Design review of the part built by this model. Coordinates are the model's own, in mm. A direction names the side the tool comes from. Coordinates: 2 decimals unless noted, no trailing zeros. Write each loop counter-clockwise with the first axis right and the second up, starting at its lowest first coordinate (ties: lowest second). Pieces come first, ordered by that corner, then holes. Notation, with made-up numbers: (3, 19) - (62, 19) arc R18 cw to (62, 30) - close; hole circle Ø7 at (85, 88). An arc over 180 degrees is marked (long way). One line per item, written item: value.
Autodesk Inventor part; units mm, degrees
ref_plane "YZ Plane" through (0, 0, 0) normal (1, 0, 0) x (0, 1, 0)
ref_plane "XZ Plane" through (0, 0, 0) normal (0, 1, 0) x (-1, 0, 0)
ref_plane "XY Plane" through (0, 0, 0) normal (0, 0, 1) x (1, 0, 0)
sketch "Sketch1" plane through (0, 0, 0) normal (0, 0, 1) x (1, 0, 0)
  line L0 (0, 0) -> (88.1, 0)
  line L1 (88.1, 0) -> (88.1, 13.5)
  line L2 (88.1, 13.5) -> (0, 13.5)
  line L3 (0, 13.5) -> (0, 0)
  dimension "d0" = 88.1
  dimension "d1" = 13.5
extrude "Extrusion1" add sketch "Sketch1" along normal blind 6
sketch "Sketch2" plane through (0, 0, 6) normal (0, 0, 1) x (1, 0, 0)
  line L0 (0, 0) -> (88.1, 0)
  line L1 (88.1, 13.5) -> (0, 13.5)
  line L2 (40.05, 13.5) -> (48.05, 13.5)
  line L3 (48.05, 13.5) -> (48.05, 17.5)
  line L4 (46.05, 19.5) -> (42.05, 19.5)
  line L5 (40.05, 17.5) -> (40.05, 13.5)
  line L6 (70.05, 13.5) -> (78.05, 13.5)
  line L7 (78.05, 13.5) -> (78.05, 17.5)
  line L8 (76.05, 19.5) -> (72.05, 19.5)
  line L9 (70.05, 17.5) -> (70.05, 13.5)
  line L10 (10.05, 13.5) -> (18.05, 13.5)
  line L11 (18.05, 13.5) -> (18.05, 17.5)
  line L12 (16.05, 19.5) -> (12.05, 19.5)
  line L13 (10.05, 17.5) -> (10.05, 13.5)
  line L14 (10.05, 0) -> (18.05, 0)
  line L15 (18.05, 0) -> (18.05, -4)
  line L16 (16.05, -6) -> (12.05, -6)
  line L17 (10.05, -4) -> (10.05, 0)
  line L18 (40.05, 0) -> (48.05, 0)
  line L19 (48.05, 0) -> (48.05, -4)
  line L20 (46.05, -6) -> (42.05, -6)
  line L21 (40.05, -4) -> (40.05, 0)
  line L22 (70.05, 0) -> (78.05, 0)
  line L23 (78.05, 0) -> (78.05, -4)
  line L24 (76.05, -6) -> (72.05, -6)
  line L25 (70.05, -4) -> (70.05, 0)
  arc A0 (12.05, 19.5) -> (10.05, 17.5) centre (12.05, 17.5) ccw
  arc A1 (18.05, 17.5) -> (16.05, 19.5) centre (16.05, 17.5) ccw
  arc A2 (42.05, 19.5) -> (40.05, 17.5) centre (42.05, 17.5) ccw
  arc A3 (48.05, 17.5) -> (46.05, 19.5) centre (46.05, 17.5) ccw
  arc A4 (72.05, 19.5) -> (70.05, 17.5) centre (72.05, 17.5) ccw
  arc A5 (78.05, 17.5) -> (76.05, 19.5) centre (76.05, 17.5) ccw
  arc A6 (70.05, -4) -> (72.05, -6) centre (72.05, -4) ccw
  arc A7 (76.05, -6) -> (78.05, -4) centre (76.05, -4) ccw
  arc A8 (40.05, -4) -> (42.05, -6) centre (42.05, -4) ccw
  arc A9 (46.05, -6) -> (48.05, -4) centre (46.05, -4) ccw
  arc A10 (16.05, -6) -> (18.05, -4) centre (16.05, -4) ccw
  arc A11 (10.05, -4) -> (12.05, -6) centre (12.05, -4) ccw
  line L26 (88.1, 13.5) -> (0, 13.5)
  line L27 (18.05, 15.5) -> (40.05, 15.5) construction
  line L28 (48.05, 15.5) -> (70.05, 15.5) construction
  point P0 (44.05, 19.5)
  point P1 (44.05, 13.5)
  dimension "d4" = 2
  dimension "d5" = 8
  dimension "d6" = 8
  dimension "d7" = 8
  dimension "d8" = 6
  dimension "d9" = 6
  dimension "d10" = 22
extrude "Extrusion2" add sketch "Sketch2" against normal blind 6
sketch "Sketch3" plane through (0, 0, 6) normal (0, 0, 1) x (1, 0, 0)
  line L0 (0, 13.5) -> (0, 0)
  circle A0 centre (31.889, 6.75) radius 2.25
  circle A1 centre (75.859, 6.75) radius 2.25
  point P0 (0, 6.75)
  dimension "d13" = 31.889
  dimension "d14" = 75.859
  dimension "d15" = 4.5
extrude "Extrusion3" cut sketch "Sketch3" against normal through all
properties part number "rope_mount_holder"
1. Consider section C-C, the plane z = 2.95. Give the number of separate pieces and of enclosed holes in the cut face, then the cut area to 3 significant figures.
Answer block:
separate pieces: 1
enclosed holes: 2
area: 1,440 mm^2
2. Wall thickness on line 1 along X through (y, z) = (-1, 4.6); line 2 along X through (y, z) = (8.5, 2.25); line 3 along Y through (x, z) = (81.5, 4.1): over which ranges is each line inside the solid? List them lowest first.
Answer block:
line 1: x = 10.05 to 18.05, 40.05 to 48.05, 70.05 to 78.05
line 2: x = 0 to 30.47, 33.3 to 74.44, 77.27 to 88.1
line 3: y = 0 to 13.5
3. Insertion check: pin 1 Ø1.2 at (y, z) = (-2, 3) entering from +X; pin 2 Ø1.8 at (x, z) = (85, 3.5) entering from -Y; pin 3 Ø3 at (y, z) = (-3, 3) entering from -X. Each pin has a flat end and moves straight along its axis. Give the tip position at first contact, or say it passes through.
Answer block:
pin 1: stops at x = 78.05
pin 2: stops at y = 0
pin 3: stops at x = 10.05
4. Consider section A-A, the plane y = 6.75. Write out the cut boundary in (x, z).
Answer block:
outline: (0, 0) - (29.64, 0) - (29.64, 6) - (0, 6) - close; (34.14, 0) - (73.61, 0) - (73.61, 6) - (34.14, 6) - close; (78.11, 0) - (88.1, 0) - (88.1, 6) - (78.11, 6) - close
5. Mouldability with a two-part tool opening along Y and no side actions: class faces 1 (the face through (74.2, 8.27, 3.04)), 2 (the face through (78.05, 15, 3)), 3 (the face through (70.62, -5.4, 3.04)), 4 (the face through (44, 19.5, 3)) as released by +Y, released by -Y, zero draft, split by the parting line, or undercut.
Answer block:
face 1: undercut
face 2: zero draft
face 3: released by -Y
face 4: released by +Y
6. Consider section B-B, the plane x = 9. Write out the cut boundary in (y, z).
Answer block:
outline: (0, 0) - (13.5, 0) - (13.5, 6) - (0, 6) - close
7. For faces 5 (the face through (78.05, -2, 3)), 6 (the face through (18.05, -2, 3)), 7 (the face through (5, 13.5, 3)), list the 3-axis set-ups (+Z, -Z, +X, -X, +Y, -Y) from which the entire face can be reached by the end or side of a thin tool; tool diameter is ignored.
Answer block:
face 5: +Z, -Z, +X, -Y
face 6: +Z, -Z, -Y
face 7: +Z, -Z, -X, +Y
